```python
from build123d import *

# Parameters (mm, degrees)
DODANIE_WYCI_GNI_CIE1_OUTLINE_R   = 1.75
DODANIE_WYCI_GNI_CIE1_OUTLINE_R_2 = 6
DODANIE_WYCI_GNI_CIE1_DEPTH       = 5
SZKIC2_W                          = 36.8
SZKIC2_H                          = 5
DODANIE_WYCI_GNI_CIE2_DEPTH       = 50
SFAZOWANIE1_SIZE                  = 10


# Read off the part's stored shape, not the designer's step: Dodanie-wyci_gni_cie1
with BuildPart() as part:
    # Dodanie-wyci_gni_cie1 outline → Dodanie-wyci_gni_cie1 (new body)
    with BuildSketch(Plane.ZY.offset(-752.608350006)):
        with BuildLine():
            Line((1104.060111381, -1919), (1104.060111381, -2000))
            Line((1104.060111381, -2000), (1140.860111381, -2000))
            Line((1140.860111381, -2000), (1140.860111381, -1919))
            ThreePointArc((1140.860111381, -1919), (1122.460111381, -1900.6), (1104.060111381, -1919))
        make_face()
        with Locations((1114.710111381, -1932.423393759)):
            Circle(DODANIE_WYCI_GNI_CIE1_OUTLINE_R, mode=Mode.SUBTRACT)
        with Locations((1122.460111381, -1926)):
            Circle(DODANIE_WYCI_GNI_CIE1_OUTLINE_R_2, mode=Mode.SUBTRACT)
        with Locations((1106.960111381, -1919)):
            Circle(DODANIE_WYCI_GNI_CIE1_OUTLINE_R, mode=Mode.SUBTRACT)
        with Locations((1114.710111381, -1905.576606241)):
            Circle(DODANIE_WYCI_GNI_CIE1_OUTLINE_R, mode=Mode.SUBTRACT)
        with Locations((1130.210111381, -1932.423393759)):
            Circle(DODANIE_WYCI_GNI_CIE1_OUTLINE_R, mode=Mode.SUBTRACT)
        with Locations((1130.210111381, -1905.576606241)):
            Circle(DODANIE_WYCI_GNI_CIE1_OUTLINE_R, mode=Mode.SUBTRACT)
        with Locations((1137.960111381, -1919)):
            Circle(DODANIE_WYCI_GNI_CIE1_OUTLINE_R, mode=Mode.SUBTRACT)
    extrude(amount=DODANIE_WYCI_GNI_CIE1_DEPTH)

    # Szkic2 → Dodanie-wyci_gni_cie2 (add)
    with BuildSketch(Plane.ZY.offset(-752.608350006)):
        with Locations((1122.460111381, -1997.5)):
            Rectangle(SZKIC2_W, SZKIC2_H)
    extrude(amount=-DODANIE_WYCI_GNI_CIE2_DEPTH)

    # Sfazowanie1
    sfazowanie1_edges = [part.edges().sort_by_distance(p)[0] for p in [
        (752.608350006, -1995, 1122.460111381),
    ]]
    chamfer(sfazowanie1_edges, length=SFAZOWANIE1_SIZE)


solid = part.part
```
Here's how the part is built. I have some questions about the finished solid (model axes, mm). A direction names the side the tool comes from. Coordinates: 2 decimals unless noted, no trailing zeros. Order: outer loops, then holes, each group sorted by start corner. A loop starts at its lowest first (then second) coordinate and runs counter-clockwise, first axis right, second up. Notation, with made-up numbers: (83.5, 41.25) - (95.5, 41.25) arc R24 cw to (95.5, 57.25) - close; hole circle Ø9 at (28, -29). An arc over 180 degrees is marked (long way). One line per question, with ' | ' between items.
(1) Will these pins go through, and if not, where does the flat tip stop? pin 1 (19 mm diameter, centred on y = -1926, z = 1122.46, fed in from +X); pin 2 (4 mm diameter, centred on y = -1919, z = 1137.96, fed in from -X).
Report:
pin 1: stops at x = 752.61 | pin 2: stops at x = 747.61
(2) If we mould it in two halves opening along Z, with no side actions, what happens to faces 3 (the cylindrical face through (750.14, -1932.35, 1112.96)), 4 (the cylindrical face through (750.143, -1931.323, 1125.229)), 5 (the flat face through (752.608, -1942, 1122)), 6 (the cylindrical face through (750.143, -1900.604, 1122.865))? For each: pulls with the +Z half, pulls with the -Z half, needs draft (parallel to the pull), parting line crosses it, or undercut.
Report:
face 3: undercut | face 4: undercut | face 5: needs draft | face 6: parting line crosses it
(3) Suppose I cut it at D-D on y = -1942. List the corners of the cut face in (x, z) for me.
Report:
outline: (747.61, 1104.06) - (752.61, 1104.06) - (752.61, 1140.86) - (747.61, 1140.86) - close
(4) For faces 1 (the flat face through (782, -1995, 1122)), 2 (the cylindrical face through (750.14, -1917.82, 1136.67)), which set-ups out of +Z, -Z, +X, -X, +Y, -Y let a thin tool reach every point of the face, with its end or its side?
Report:
face 1: +Z, -Z, +X, +Y | face 2: +X, -X
(5) Suppose I cut it at C-C on z = 1115. List the corners of the cut face in (x, y) for me, and give its area (3 significant figures).
Report:
outline: (747.61, -2000) - (802.61, -2000) - (802.61, -1995) - (762.61, -1995) - (752.61, -1985) - (752.61, -1934.15) - (747.61, -1934.15) - close; (747.61, -1930.7) - (752.61, -1930.7) - (752.61, -1907.3) - (747.61, -1907.3) - close; (747.61, -1903.85) - (752.61, -1903.85) - (752.61, -1902.18) - (747.61, -1902.18) - close | area: 755 mm2
(6) Suppose I cut it at A-A on z = 1123. List the corners of the cut face in (x, y) for me, and give its area (3 significant figures).
Report:
outline: (747.61, -2000) - (802.61, -2000) - (802.61, -1995) - (762.61, -1995) - (752.61, -1985) - (752.61, -1931.98) - (747.61, -1931.98) - close; (747.61, -1920.02) - (752.61, -1920.02) - (752.61, -1900.61) - (747.61, -1900.61) - close | area: 737 mm2
(7) Suppose I cut it at B-B on y = -1926. List the corners of the cut face in (x, z) for me, and give its area (3 significant figures).
Report:
outline: (747.61, 1104.06) - (752.61, 1104.06) - (752.61, 1116.46) - (747.61, 1116.46) - close; (747.61, 1128.46) - (752.61, 1128.46) - (752.61, 1140.86) - (747.61, 1140.86) - close | area: 124 mm2
(8) If I drill on L1, parallel to Z at x = 749.65, y = -1919; L2, parallel to Y at x = 763, z = 1118; L3, parallel to X at y = -1936.5, z = 1132, over which ranges is the centre line in solid material (lowest first)?
Report:
L1: z = 1104.06 to 1105.21, 1108.71 to 1136.21, 1139.71 to 1140.86 | L2: y = -2000 to -1995 | L3: x = 747.61 to 752.61
